The listing builds one solid part. Answer for the finished solid, in the listing's coordinates (mm). A direction names the side the tool comes from. Give positions to 0.01 mm unless a question says otherwise; leave off trailing zeros. Write each loop counter-clockwise with the first axis right and the second up, starting at its lowest first coordinate (ties: lowest second). Pieces come first, ordered by that corner, then holes. Notation, with made-up numbers: (27.5, 86.5) -> (66.5, 86.5) arc R36 ccw to (66.5, 120.5) -> close; hole circle Ø5 at (14.25, 48.25). An arc over 180 degrees is marked (long way). One line per question, with ' | ' between items.
from build123d import *

# Parameters (mm, degrees)
SKETCH008_W     = 90
SKETCH008_H     = 150
PAD003_DEPTH    = 35
SKETCH009_W     = 81
SKETCH009_H     = 141
POCKET003_DEPTH = 30.5
SKETCH013_R     = 5.5
PAD006_DEPTH    = 150
SKETCH014_W     = 51
SKETCH014_H     = 14
POCKET005_DEPTH = 6
PAD008_DEPTH    = 49.5
PAD009_DEPTH    = 49.5
SKETCH021_W     = 20
SKETCH021_H     = 6.65
PAD010_DEPTH    = 51
CHAMFER001_SIZE = 15
SKETCH022_R     = 0.75
POCKET007_DEPTH = 11.8
CHAMFER002_SIZE = 16
CHAMFER003_SIZE = 9
FILLET001_R     = 24
SKETCH023_W     = 6.5
SKETCH023_H     = 25.5
POCKET008_DEPTH = 16


with BuildPart() as part:
    # Sketch008 → Pad003 (new body)
    with BuildSketch(Plane.XY):
        with Locations((45, 75)):
            Rectangle(SKETCH008_W, SKETCH008_H)
    extrude(amount=PAD003_DEPTH)

    # Sketch009 (on Face6 of Pad003) → Pocket003 (cut)
    with BuildSketch(Plane.XY.offset(35)):
        with Locations((45, 75)):
            Rectangle(SKETCH009_W, SKETCH009_H)
    extrude(amount=-POCKET003_DEPTH, mode=Mode.SUBTRACT)

    # Sketch013 → Pad006 (join)
    with BuildSketch(Plane.XZ):
        with Locations((-0.5, 35)):
            Circle(SKETCH013_R)
    extrude(amount=-PAD006_DEPTH)

    # Sketch014 → Pocket005 (cut, symmetric)
    with BuildSketch(Plane.YZ):
        with Locations((75, 33.5)):
            Rectangle(SKETCH014_W, SKETCH014_H)
    extrude(amount=POCKET005_DEPTH, both=True, mode=Mode.SUBTRACT)

    # Sketch017 (on Face13 of Pocket005) → Pad008 (join)
    with BuildSketch(Plane.XZ):
        Polygon((0, 26.7), (-6, 32.7), (-6, 35), (0, 35), align=None)
    extrude(amount=-PAD008_DEPTH)

    # Sketch018 (on Face19 of Pad008) → Pad009 (join)
    with BuildSketch(Plane.XZ.offset(-100.5)):
        Polygon((0, 26.7), (0, 35), (-6, 35), (-6, 32.7), align=None)
    extrude(amount=-PAD009_DEPTH)

    # Sketch019 (on DatumPlane) → Revolution (revolve)
    with BuildSketch(Plane(origin=(-0.5, 100.5, 0), x_dir=(0, 1, 0), z_dir=(1, 0, 0))):
        Polygon((0, 35), (-5.5, 35), (0, 29.5), align=None)
        Polygon((-51, 35), (-45.5, 35), (-51, 29.5), align=None)
    revolve(axis=Axis((-0.5, 100.5, 35), (0, -1, 0)))

    # Sketch021 (on Face26 of Revolution) → Pad010 (join)
    with BuildSketch(Plane.XY.offset(4.5)):
        with Locations((45, 120.775)):
            Rectangle(SKETCH021_W, SKETCH021_H)
        with Locations((45, 73.325)):
            Rectangle(SKETCH021_W, SKETCH021_H)
    extrude(amount=PAD010_DEPTH)

    # Chamfer001
    chamfer001_edges = [part.edges().sort_by_distance(p)[0] for p in [
        (45, 70, 4.5),
        (45, 124.1, 4.5),
    ]]
    chamfer(chamfer001_edges, length=CHAMFER001_SIZE)

    # Sketch022 (on Face23 of Chamfer001) → Pocket007 (cut)
    with BuildSketch(Plane.XY.offset(55.5)):
        with Locations((39, 121)):
            Circle(SKETCH022_R)
        with Locations((51, 121)):
            Circle(SKETCH022_R)
        with Locations((39, 73)):
            Circle(SKETCH022_R)
        with Locations((51, 73)):
            Circle(SKETCH022_R)
    extrude(amount=-POCKET007_DEPTH, mode=Mode.SUBTRACT)

    # Chamfer002
    chamfer002_edges = [part.edges().sort_by_distance(p)[0] for p in [
        (45, 70, 19.5),
        (45, 124.1, 19.5),
    ]]
    chamfer(chamfer002_edges, length=CHAMFER002_SIZE)

    # Chamfer003
    chamfer003_edges = [part.edges().sort_by_distance(p)[0] for p in [
        (45, 70, 35.5),
        (45, 124.1, 35.5),
    ]]
    chamfer(chamfer003_edges, length=CHAMFER003_SIZE)

    # Fillet001
    fillet001_edges = [part.edges().sort_by_distance(p)[0] for p in [
        (45, 124.1, 44.5),
        (45, 127.544151, 27.185084),
        (45, 135.413708, 8.186292),
        (45, 58.686292, 8.186292),
        (45, 66.555849, 27.185084),
        (45, 70, 44.5),
    ]]
    fillet(fillet001_edges, radius=FILLET001_R)

    # Sketch023 (on Face6 of Fillet001) → Pocket008 (cut)
    with BuildSketch(Plane(origin=(0, 76.65, 0), x_dir=(-1, 0, 0), z_dir=(0, 1, 0))):
        with Locations((-45, 42.75)):
            Rectangle(SKETCH023_W, SKETCH023_H)
    extrude(amount=-POCKET008_DEPTH, mode=Mode.SUBTRACT)


solid = part.part
Item 1: Flat-ended cylindrical pins translate along their axes: pin 1 (3.5 mm diameter, centred on x = 51.5, z = 50.5, fed in from -Y); pin 2 (5 mm diameter, centred on x = 45.5, y = 70.5, fed in from +Z); pin 3 (6 mm diameter, centred on x = 72.5, z = 21.5, fed in from -Y); pin 4 (1 mm diameter, centred on x = 44.5, z = 46.5, fed in from +Y). Find the tip coordinate at first contact, or state that the pin passes through.
Answers below:
pin 1: y = 70 | pin 2: z = 30 | pin 3: y = 0 | pin 4: y = 124.12
Item 2: Find section A-A (y = 99). Write down the section's boundary in (x, z), then the cut area to 3 significant figures.
Answers below:
outline: circle Ø8 at (-0.5, 35); (0, 0) -> (90, 0) -> (90, 35) -> (85.5, 35) -> (85.5, 4.5) -> (4.5, 4.5) -> (4.5, 26.5) -> (0, 26.5) -> close | area: 692 mm²
Item 3: Find section D-D (y = 81.5). Write down the section's boundary in (x, z), then the cut area to 3 significant figures.
Answers below:
outline: (0, 0) -> (90, 0) -> (90, 35) -> (85.5, 35) -> (85.5, 4.5) -> (4.5, 4.5) -> (4.5, 26.5) -> (0, 26.5) -> close | area: 641 mm²
Item 4: Find section B-B (z = 23.5). Write down the section's boundary in (x, y).
Answers below:
outline: (0, 0) -> (90, 0) -> (90, 150) -> (0, 150) -> close; (35, 65.03) -> (55, 65.03) -> (55, 76.65) -> (35, 76.65) -> close; (35, 117.45) -> (55, 117.45) -> (55, 129.07) -> (35, 129.07) -> close; hole (4.5, 4.5) -> (85.5, 4.5) -> (85.5, 145.5) -> (4.5, 145.5) -> close
Item 5: Find section C-C (x = 16.5). Write down the section's boundary in (y, z), then the cut area to 4 significant figures.
Answers below:
outline: (0, 0) -> (150, 0) -> (150, 35) -> (145.5, 35) -> (145.5, 4.5) -> (4.5, 4.5) -> (4.5, 35) -> (0, 35) -> close | area: 949.5 mm²
Item 6: Determine the mould class of faces 1 (the face through (45, 124.1, 51)), 2 (the face through (-3, 124.9, 29.7)), 3 (the face through (55, 123, 24)) for opening direction X: pulls with the +X half, pulls with the -X half, needs draft (parallel to the pull), parting line crosses it, or undercut.
Answers below:
face 1: needs draft | face 2: pulls with the -X half | face 3: undercut
Item 7: Consider line 1 (X direction, y = 73, z = 50); line 2 (Y direction, x = 51, z = 49); line 3 (X direction, y = 121, z = 47). Determine where each line is inside the solid, lowest interval first. Write a range as [from, to].
Answers below:
line 1: [35, 38.25], [39.75, 41.75], [48.25, 50.25], [51.75, 55] | line 2: [70, 72.25], [73.75, 76.65], [117.45, 120.25], [121.75, 124.1] | line 3: [35, 38.25], [39.75, 50.25], [51.75, 55]
Item 8: A tool of negligible diameter and unlimited length cuts with its end or side. For faces 4 (the face through (45, 121, 55.5)), 5 (the face through (44.86, 130.98, 18.89)), 6 (the face through (2, 100.5, 29)), from which of +Z, -Z, +X, -X, +Y, -Y can it reach the whole face along a straight path? Write none if from no direction.
Answers below:
face 4: +Z, +X, -X, +Y, -Y | face 5: +Z | face 6: none
